from build123d import *

# Parameters (mm, degrees)
SKETCH_W     = 53
SKETCH_H     = 80
PAD_DEPTH    = 1
SKETCH001_R  = 1.5
PAD001_DEPTH = 2.5
SKETCH002_R  = 2.5
PAD002_DEPTH = 1


with BuildPart() as part:
    # Sketch → Pad (new body)
    with BuildSketch(Plane.XY):
        Rectangle(SKETCH_W, SKETCH_H)
    extrude(amount=PAD_DEPTH)

    # Sketch001 (on Face6 of Pad) → Pad001 (join)
    with BuildSketch(Plane.XY.offset(1)):
        with Locations((0, 21.5)):
            Circle(SKETCH001_R)
        with Locations((0, -21.5)):
            Circle(SKETCH001_R)
    extrude(amount=PAD001_DEPTH)

    # Sketch002 (on Face9 of Pad001) → Pad002 (join)
    with BuildSketch(Plane.XY.offset(3.5)):
        with Locations((0, 21.5)):
            Circle(SKETCH002_R)
        with Locations((0, -21.5)):
            Circle(SKETCH002_R)
    extrude(amount=PAD002_DEPTH)


solid = part.part
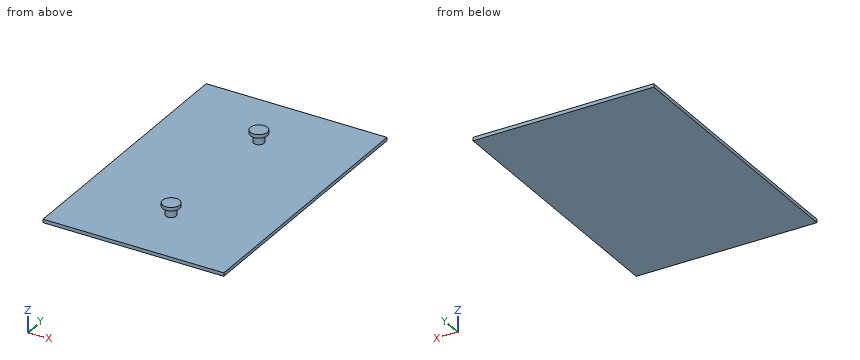
Geometry: final body of the model. Coordinates: model frame, mm. Coordinates: 2 decimals unless noted, no trailing zeros. Order: outer loops, then holes, each group sorted by start corner. A loop starts at its lowest first (then second) coordinate and runs counter-clockwise, first axis right, second up.
(1) First-contact query: pin 1 (5 mm diameter, centred on x = -17.5, y = 18.5, fed in from +Z). Flat tip, straight axial feed; report the tip coordinate or a pass-through.
(2) Section query B-B (y = 21.5). Return the cut outline in (x, z), plus the area to 3 significant figures.
(3) Section query D-D (y = -9.5). Return the cut outline in (x, z), plus the area to 3 significant figures.
(4) Section query A-A (x = 0). Return the cut outline in (y, z), plus the area to 3 significant figures.
(5) Material intervals for probe 1 along Z at (x, y) = (-10, -33); probe 2 along Y at (x, z) = (1, 1.8), sorted ascending.
(6) Section query C-C (x = -12.5). Return the cut outline in (y, z).
Solution:
1. pin 1: stops at z = 1
2. outline: (-26.5, 0) - (26.5, 0) - (26.5, 1) - (1.5, 1) - (1.5, 3.5) - (2.5, 3.5) - (2.5, 4.5) - (-2.5, 4.5) - (-2.5, 3.5) - (-1.5, 3.5) - (-1.5, 1) - (-26.5, 1) - close
2. area: 65.5 mm2
3. outline: (-26.5, 0) - (26.5, 0) - (26.5, 1) - (-26.5, 1) - close
3. area: 53.0 mm2
4. outline: (-40, 0) - (40, 0) - (40, 1) - (23, 1) - (23, 3.5) - (24, 3.5) - (24, 4.5) - (19, 4.5) - (19, 3.5) - (20, 3.5) - (20, 1) - (-20, 1) - (-20, 3.5) - (-19, 3.5) - (-19, 4.5) - (-24, 4.5) - (-24, 3.5) - (-23, 3.5) - (-23, 1) - (-40, 1) - close
4. area: 105 mm2
5. probe 1: z = 0 to 1
5. probe 2: y = -22.62 to -20.38, 20.38 to 22.62
6. outline: (-40, 0) - (40, 0) - (40, 1) - (-40, 1) - close
